from build123d import *

# Parameters (mm, degrees)
BOSS_EXTRUDE1_DEPTH = 1.5875
SKETCH5_R           = 2.2098
CUT_EXTRUDE1_DEPTH  = 2.5875


with BuildPart() as part:
    # Sketch4 → Boss-Extrude1 (new body)
    with BuildSketch(Plane(origin=(0, 0, 0), x_dir=(1, 0, 0), z_dir=(0, 1, 0))):
        with BuildLine():
            Line((-29.21, 76.2), (29.21, 76.2))
            ThreePointArc((29.21, 76.2), (31.006051224, 75.456051224), (31.75, 73.66))
            Line((31.75, 73.66), (31.75, 40.64))
            ThreePointArc((31.75, 40.64), (31.006051224, 38.843948776), (29.21, 38.1))
            Line((29.21, 38.1), (26.67, 38.1))
            ThreePointArc((26.67, 38.1), (21.59, 33.02), (26.67, 27.94))
            Line((26.67, 27.94), (29.21, 27.94))
            ThreePointArc((29.21, 27.94), (31.006051224, 27.196051224), (31.75, 25.4))
            Line((31.75, 25.4), (31.75, -17.78))
            ThreePointArc((31.75, -17.78), (31.006051224, -19.576051224), (29.21, -20.32))
            Line((29.21, -20.32), (-29.21, -20.32))
            ThreePointArc((-29.21, -20.32), (-31.006051224, -19.576051224), (-31.75, -17.78))
            Line((-31.75, -17.78), (-31.75, 25.4))
            ThreePointArc((-31.75, 25.4), (-31.006051224, 27.196051224), (-29.21, 27.94))
            Line((-29.21, 27.94), (-26.67, 27.94))
            ThreePointArc((-26.67, 27.94), (-21.59, 33.02), (-26.67, 38.1))
            Line((-26.67, 38.1), (-29.21, 38.1))
            ThreePointArc((-29.21, 38.1), (-31.006051224, 38.843948776), (-31.75, 40.64))
            Line((-31.75, 40.64), (-31.75, 73.66))
            ThreePointArc((-31.75, 73.66), (-31.006051224, 75.456051224), (-29.21, 76.2))
        make_face()
    extrude(amount=-BOSS_EXTRUDE1_DEPTH)

    # Sketch5 → Cut-Extrude1 (cut, through all)
    with BuildSketch(Plane(origin=(0, 0, 0), x_dir=(1, 0, 0), z_dir=(0, 1, 0))):
        with Locations((-27.94, 72.39)):
            Circle(SKETCH5_R)
        with Locations((27.94, 72.39)):
            Circle(SKETCH5_R)
        with Locations((-27.94, -16.51)):
            Circle(SKETCH5_R)
        with Locations((27.94, -16.51)):
            Circle(SKETCH5_R)
        with Locations((-27.94, 16.51)):
            Circle(SKETCH5_R)
        with Locations((27.94, 16.51)):
            Circle(SKETCH5_R)
    extrude(amount=-CUT_EXTRUDE1_DEPTH, mode=Mode.SUBTRACT)


solid = part.part
Geometry check sheet. Reference: the model listing, model coordinates, mm. A direction names the side the tool comes from. Coordinates: 2 decimals unless noted, no trailing zeros. Order: outer loops, then holes, each group sorted by start corner. A loop starts at its lowest first (then second) coordinate and runs counter-clockwise, first axis right, second up. Notation, with made-up numbers: (53.5, 10) -> (78.5, 10) arc R27 ccw to (78.5, 41) -> close; hole circle Ø1 at (11, 41). An arc over 180 degrees is marked (long way). Use a Markdown table: item, result. Add a question column.
1. Cross-section at B-B (z = 16.51). Enter the section's corners in (x, y), and give its area (3 significant figures).
2. Cross-section at A-A (x = 27.94). Enter the section's corners in (y, z).
3. Go/stop test with a flat-tipped pin: pin 1 Ø4 at (x, z) = (27.94, -16.51) entering from -Y. Record where the tip stops, or that it passes through.
4. Set-up check for faces 1 (the face through (-31, -0.8, -27.2)), 2 (the face through (30.986, -0.783, -75.476)), 3 (the face through (31, -0.8, -27.2)): record each of +Z, -Z, +X, -X, +Y, -Y from which the full face is reachable in a straight line by a thin tool's end or side.
5. Material ranges on L1, parallel to X at y = -1.05, z = -72.39; L2, parallel to Z at x = 27.94, y = -0.6; L3, parallel to Z at x = 27, y = -1.1, recorded low to high.
6. Cross-section at C-C (y = -1.05). Enter the section's corners in (x, z).
7. Mould release check, pull along X, two halves, no side actions. Record for faces 4 (the face through (-29.57, -0.78, -73.88)), 5 (the face through (-29.694, -0.783, 17.855)), 6 (the face through (21.59, -0.78, -33.13)), 7 (the face through (-31.026, -0.783, -75.436)): pulls with the +X half, pulls with the -X half, needs draft (parallel to the pull), parting line crosses it, or undercut.
Filled sheet:
| question | item | result |
|---|---|---|
| 1 | outline | (-31.75, -1.59) -> (-30.15, -1.59) -> (-30.15, 0) -> (-31.75, 0) -> close; (-25.73, -1.59) -> (25.73, -1.59) -> (25.73, 0) -> (-25.73, 0) -> close; (30.15, -1.59) -> (31.75, -1.59) -> (31.75, 0) -> (30.15, 0) -> close |
| 1 | area | 86.8 mm2 |
| 2 | outline | (-1.59, -76.2) -> (0, -76.2) -> (0, -74.6) -> (-1.59, -74.6) -> close; (-1.59, -70.18) -> (0, -70.18) -> (0, -38.1) -> (-1.59, -38.1) -> close; (-1.59, -27.94) -> (0, -27.94) -> (0, -18.72) -> (-1.59, -18.72) -> close; (-1.59, -14.3) -> (0, -14.3) -> (0, 14.3) -> (-1.59, 14.3) -> close; (-1.59, 18.72) -> (0, 18.72) -> (0, 20.32) -> (-1.59, 20.32) -> close |
| 3 | pin 1 | through |
| 4 | face 1 | -X, +Y, -Y |
| 4 | face 2 | -Z, +X, +Y, -Y |
| 4 | face 3 | +X, +Y, -Y |
| 5 | L1 | -31.75 to -30.15, -25.73 to 25.73, 30.15 to 31.75 |
| 5 | L2 | -76.2 to -74.6, -70.18 to -38.1, -27.94 to -18.72, -14.3 to 14.3, 18.72 to 20.32 |
| 5 | L3 | -76.2 to -74.39, -70.39 to -38.1, -27.94 to -18.51, -14.51 to 14.51, 18.51 to 20.32 |
| 6 | outline | (-31.75, -73.66) arc R2.54 ccw to (-29.21, -76.2) -> (29.21, -76.2) arc R2.54 ccw to (31.75, -73.66) -> (31.75, -40.64) arc R2.54 ccw to (29.21, -38.1) -> (26.67, -38.1) arc R5.08 cw to (26.67, -27.94) -> (29.21, -27.94) arc R2.54 ccw to (31.75, -25.4) -> (31.75, 17.78) arc R2.54 ccw to (29.21, 20.32) -> (-29.21, 20.32) arc R2.54 ccw to (-31.75, 17.78) -> (-31.75, -25.4) arc R2.54 ccw to (-29.21, -27.94) -> (-26.67, -27.94) arc R5.08 cw to (-26.67, -38.1) -> (-29.21, -38.1) arc R2.54 ccw to (-31.75, -40.64) -> close; hole circle Ø4.42 at (-27.94, -72.39); hole circle Ø4.42 at (-27.94, -16.51); hole circle Ø4.42 at (-27.94, 16.51); hole circle Ø4.42 at (27.94, -72.39); hole circle Ø4.42 at (27.94, -16.51); hole circle Ø4.42 at (27.94, 16.51) |
| 7 | face 4 | undercut |
| 7 | face 5 | undercut |
| 7 | face 6 | pulls with the +X half |
| 7 | face 7 | pulls with the -X half |
